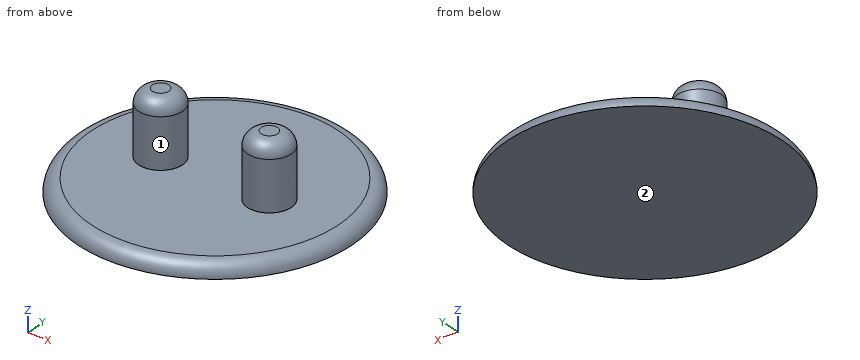
```python
from build123d import *

# Parameters (mm, degrees)
F0_R     = 10
F0_R_2   = 1.6
F1_DEPTH = 1
F2_DEPTH = 4.6
F3_R     = 1
F4_R     = 0.99999


# Not quite as in the source:
# - a fillet or chamfer is up to 0.001 mm smaller than in the source, because OpenCascade refuses the exact size


with BuildPart() as f1:
    # F0 (on Top) → F1 (new body)
    with BuildSketch(Plane.XY):
        Circle(F0_R)
        with Locations((-4, 0)):
            Circle(F0_R_2, mode=Mode.SUBTRACT)
        with Locations((4, 0)):
            Circle(F0_R_2, mode=Mode.SUBTRACT)
        with Locations((-4, 0)):
            Circle(F0_R_2)
        with Locations((4, 0)):
            Circle(F0_R_2)
    extrude(amount=-F1_DEPTH)

    # F0 (on Top) → F2 (join)
    with BuildSketch(Plane.XY):
        with Locations((-4, 0)):
            Circle(F0_R_2)
        with Locations((4, 0)):
            Circle(F0_R_2)
    extrude(amount=F2_DEPTH)

    # F3
    f3_edges = [f1.edges().sort_by_distance(p)[0] for p in [
        (-5.6, 0, 4.6),
        (2.4, 0, 4.6),
    ]]
    fillet(f3_edges, radius=F3_R)

    # F4 (radius 1 in the source; OpenCascade refuses exactly that, so slightly less here)
    f4_edges = [f1.edges().sort_by_distance(p)[0] for p in [
        (-10, 0, 0),
    ]]
    fillet(f4_edges, radius=F4_R)


solid = f1.part
```
The model under review builds one solid part; all positions refer to its coordinate system, in mm. Face numbers are marked on the shaded views. Round coordinates to 2 decimals unless told otherwise and drop trailing zeros. Write each loop counter-clockwise with the first axis right and the second up, starting at its lowest first coordinate (ties: lowest second). Pieces come first, ordered by that corner, then holes. Notation, with made-up numbers: M -40,27 L 9,27 A5 ccw 9,31 Z; hole C 20.5,-32 d2. An arc over 180 degrees is marked long. Use CSV: the item, a comma, the result in double quotes. Start each with the question number.
(1) Clearance check with flat-ended pins moving along their axes: P1, Ø1.5, axis at y = -7.5, z = 1, coming from the -X side; P2, Ø6, axis at x = 6.5, y = 8, coming from the +Z side; P3, Ø5.5, axis at x = 3, y = 0.5, coming from the +Z side. State where each tip first meets the part, or that it passes through.
(2) The part is to be moulded in two halves that separate along X. For the marked faces 1 and 2, say which applies: +X half, -X half, draft (parallel to the pull), parting line (faces both ways), or undercut.
(3) For line 1 along Z through (x, y) = (1.5, 2); line 2 along Y through (x, z) = (-9, -0.4); line 3 along Y through (x, z) = (-3.25, 2.9), list the stretches that pass through material, from the lowest coordinate up.
(4) We need section A-A, the plane z = 1.25. State the section outline as (x, y) points, then the cut area to 3 significant figures.
Findings:
1,P1,"through"
1,P2,"z = 0"
1,P3,"z = 4.6"
2,face 1,"undercut"
2,face 2,"draft"
3,line 1,"-1 to 0"
3,line 2,"-3.88 to 3.88"
3,line 3,"-1.41 to 1.41"
4,outline,"C -4,0 d3.2; C 4,0 d3.2"
4,area,"16.1 mm^2"
